Part model, mm, in its own coordinate system. A direction names the side the tool comes from. Round coordinates to 2 decimals unless told otherwise and drop trailing zeros. Loops run counter-clockwise (first coordinate to the right, second up) from the corner with the lowest first, then second, coordinate; pieces in that order, holes last.
1) Band-saw the part on C-C, the plane z = 53. Write the cut outline in (x, y), then the cut area to 3 significant figures.
2) Probe line 1 (X direction, y = -18, z = 12.5); line 2 (Y direction, x = -127, z = 0); line 3 (Z direction, x = -83, y = -22). List the from-to ranges inside material, lowest first.
3) 3-axis set-ups, long thin cutter, end or side, ignore diameter. For faces 4 (the cylindrical face through (-128.54, -47.78, -2.85)), 5 (the flat face through (-141.889, -36.557, 7.035)), 6 (the flat face through (-87.16, -29.46, 45.25)), 7 (the flat face through (-129, -51.565, 3)), 8 (the flat face through (-129, -44.165, 3)): which of +Z, -Z, +X, -X, +Y, -Y reach the whole face in a straight line?
4) Band-saw the part on A-A, the plane y = -26. Write the cut outline in (x, z).
5) Mould opens along X. For faces 1 (the flat face through (-147, -35.565, 7)), 2 (the flat face through (-119.41, -46, 2)), 3 (the cylindrical face through (-96, -33, 58)) say: +X half, -X half, draft (parallel to the pull), parting line (faces both ways), or undercut.
6) Drop flat-ended pins along their axis: P1, Ø3, axis at y = -47.87, z = 0.85, coming from the +X side; P2, Ø2, axis at y = -28.5, z = 43.5, coming from the -X side; P3, Ø14.5, axis at x = -124.5, y = -40, coming from the +Z side; P4, Ø12, axis at x = -120, y = -39, coming from the -Z side. Give the stop position or say it passes through.
7) Band-saw the part on D-D, the plane z = 20. Write the cut outline in (x, y).
8) Band-saw the part on B-B, the plane x = -136. Write the cut outline in (y, z), then the cut area to 3 significant figures.
from build123d import *

# Parameters (mm, degrees)
PAD018_DEPTH    = 35
SKETCH027_R     = 2
POCKET014_DEPTH = 5
PAD019_DEPTH    = 5
SKETCH029_R     = 2
PAD020_DEPTH    = 18
POCKET015_DEPTH = 81


with BuildPart() as part:
    # Sketch026 → Pad018 (new body)
    with BuildSketch(Plane.YZ):
        with BuildLine():
            Line((-16, 30), (-34.2839170823, 65.5766549317))
            Line((-38.7309989488, 63.2911652964), (-34.2839170823, 65.5766549317))
            Line((-20.4470818665, 27.7145103647), (-38.7309989488, 63.2911652964))
            ThreePointArc((-31.5652664778, 9.5), (-20.8954209204, 15.4876380739), (-20.4470818665, 27.7145103647))
            Line((-53.5652664778, 9.5), (-31.5652664778, 9.5))
            Line((-53.5652664778, 4.5), (-53.5652664778, 9.5))
            Line((-31.5652664778, 4.5), (-53.5652664778, 4.5))
            ThreePointArc((-31.5652664778, 4.5), (-16.627666934, 12.8825899147), (-16, 30))
        make_face()
    extrude(amount=PAD018_DEPTH)

    # Sketch027 (on Face1 of Pad018) → Pocket014 (cut)
    with BuildSketch(Plane(origin=(0, -0.4604723456, -0.2366506407), x_dir=(0, -0.4570979271, 0.8894163733), z_dir=(0, 0.8894163733, 0.4570979271))):
        with Locations((41.942359, 26.427487)):
            Circle(SKETCH027_R)
        with Locations((66.942359, 26.427487)):
            Circle(SKETCH027_R)
        with Locations((66.942359, 6.427487)):
            Circle(SKETCH027_R)
        with Locations((41.942359, 6.427487)):
            Circle(SKETCH027_R)
    extrude(amount=-POCKET014_DEPTH, mode=Mode.SUBTRACT)

    # Sketch028 (on Face13 of Pocket014) → Pad019 (join)
    with BuildSketch(Plane(origin=(0, 0, 9.5), x_dir=(0, -1, 0), z_dir=(0, 0, 1))):
        with BuildLine():
            Line((53.5652664778, 0), (31.5652664778, 0))
            ThreePointArc((37.5221000572, -36), (41.5454869398, -16.8414283547), (31.5652664778, 0))
            Line((37.5221000572, -36), (35.5652664778, -39))
            Line((35.5652664778, -39), (35.5652664778, -46))
            Line((35.5652664778, -46), (53.5652664778, -46))
            Line((53.5652664778, -46), (53.5652664778, 0))
        make_face()
    extrude(amount=-PAD019_DEPTH)

    # Sketch029 (on Face15 of Pad019) → Pad020 (join)
    with BuildSketch(Plane(origin=(-33, 0, 0), x_dir=(0, 1, 0), z_dir=(-1, 0, 0))):
        with BuildLine():
            Line((-44.1652664778, -4.5), (-44.1652664778, -0.85))
            ThreePointArc((-44.1652664778, -0.85), (-47.8652664778, 2.85), (-51.5652664778, -0.85))
            Line((-51.5652664778, -4.5), (-51.5652664778, -0.85))
            Line((-51.5652664778, -4.5), (-44.1652664778, -4.5))
        make_face()
        with Locations((-47.8652664778, -0.85)):
            Circle(SKETCH029_R, mode=Mode.SUBTRACT)
    extrude(amount=-PAD020_DEPTH)

    # Sketch030 (on Face18 of Pad020) → Pocket015 (cut)
    with BuildSketch(Plane(origin=(-46, 0, 0), x_dir=(0, 1, 0), z_dir=(-1, 0, 0))):
        Polygon((-53.5652664778, -6), (-52.0652664778, -6.8660254038), (-52.0652664778, -7.1339745962), (-53.5652664778, -8), align=None)
        Polygon((-50.0652664778, -9.5), (-50.9312918816, -8), (-51.199241074, -8), (-52.0652664778, -9.5), align=None)
        Polygon((-45.699241, -8), (-46.565266, -9.5), (-44.565266, -9.5), (-45.431292, -8), align=None)
    extrude(amount=-POCKET015_DEPTH, mode=Mode.SUBTRACT)


with BuildPart() as part_1:
    # Body006 placement: moved
    add(part.part.moved(Location((-104.41, 0, 0))))


solid = part_1.part
Reported:
1. outline: (-104.41, -33.44) - (-69.41, -33.44) - (-69.41, -27.82) - (-104.41, -27.82) - close
1. area: 197 mm2
2. line 1: x = -104.41 to -69.41
2. line 2: y = -51.47 to -49.68, -46.05 to -44.26
2. line 3: z = 7.35 to 13.95, 30.74 to 41.67
3. face 4: -Z, +X, -X
3. face 5: +Z, -Z, +Y
3. face 6: +X, -X, -Y
3. face 7: -Z, +X, -X, -Y
3. face 8: -Z, +X, -X, +Y
4. outline: (-104.41, 5.41) - (-69.41, 5.41) - (-69.41, 10.81) - (-104.41, 10.81) - close; (-104.41, 38.52) - (-69.41, 38.52) - (-69.41, 49.46) - (-104.41, 49.46) - close
5. face 1: draft
5. face 2: +X half
5. face 3: undercut
6. P1: passes through
6. P2: stops at x = -104.41
6. P3: stops at z = 9.5
6. P4: stops at z = -1.49
7. outline: (-104.41, -19.23) - (-69.41, -19.23) - (-69.41, -14.18) - (-104.41, -14.18) - close
8. outline: (-53.57, 4.5) - (-51.57, 4.5) - (-51.57, 0.85) arc R3.7 ccw to (-44.17, 0.85) - (-44.17, 4.5) - (-39.85, 4.5) - (-39.85, 9.5) - (-44.57, 9.5) - (-45.43, 8) - (-45.7, 8) - (-46.57, 9.5) - (-50.07, 9.5) - (-50.93, 8) - (-51.2, 8) - (-52.07, 9.5) - (-53.57, 9.5) - (-53.57, 8) - (-52.07, 7.13) - (-52.07, 6.87) - (-53.57, 6) - close; hole circle Ø4 at (-47.87, 0.85)
8. area: 99.4 mm2
